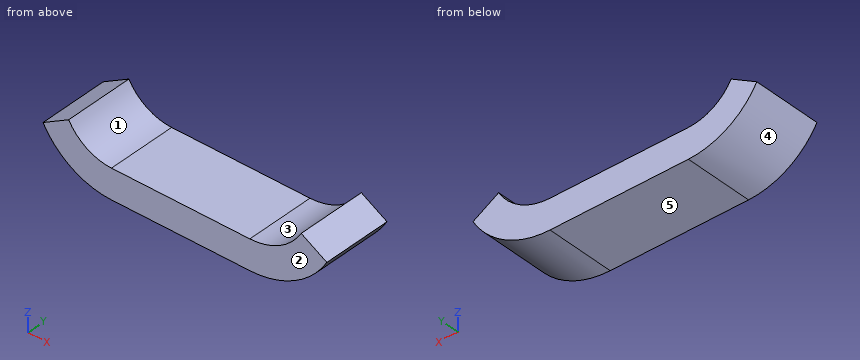
Autodesk Inventor part; units mm, degrees
ref_plane "YZ Plane" through (0, 0, 0) normal (1, 0, 0) x (0, 1, 0)
ref_plane "XZ Plane" through (0, 0, 0) normal (0, 1, 0) x (-1, 0, 0)
ref_plane "XY Plane" through (0, 0, 0) normal (0, 0, 1) x (1, 0, 0)
sketch "スケッチ1" plane through (0, 0, 0) normal (0, 1, 0) x (-1, 0, 0)
  circle A0 centre (70, -20) radius 80
  circle A1 centre (-70, -10) radius 90
  line L0 (70, -100) -> (-70, -100)
  line L1 (70, -20) -> (70, -100)
  line L2 (70, -20) -> (139.282, -60)
  line L3 (-70, -10) -> (-70, -100)
  line L4 (-70, -10) -> (-147.9423, -55)
  circle A2 centre (70, -20) radius 50
  circle A3 centre (-70, -10) radius 60
  line L5 (70, -70) -> (-70, -70)
  point P0 (0, 0)
  point P1 (113.3013, -45)
  point P2 (-121.9615, -40)
  dimension "d7" = 100
  dimension "d8" = 120
  dimension "d0" = 160
  dimension "d1" = 180
  dimension "d2" = 100
  dimension "d3" = 70
  dimension "d4" = 70
  dimension "d5" = 60
  dimension "d6" = 60
extrude "押し出し1" add sketch "スケッチ1" along normal mid plane 70 contours L1 A2 L2 A0 | L0 A1 L5 A0 | A0 L5 L1 | L3 L5 A1 | A1 L4 A3 L3
fillet "フィレット1" [suppressed]
properties part number "ArcSole2b"
Verification items for the finished model (mm, model axes). Face numbers are marked on the shaded views. A direction names the side the tool comes from. Give positions to 0.01 mm unless a question says otherwise; leave off trailing zeros. Order: outer loops, then holes, each group sorted by start corner. A loop starts at its lowest first (then second) coordinate and runs counter-clockwise, first axis right, second up. Notation, with made-up numbers: M -17.75,48.5 L 28.25,48.5 A6 cw 28.25,56.5 Z; hole C 58,80 d8. An arc over 180 degrees is marked long. Return JSON: item names as keys, results as strings. Group by question number.
1) Section check B-B on y = 17.5. Record the cut outline in (x, z), and give its area (3 significant figures).
2) Section check D-D on z = -73.5. Record the cut outline in (x, y), and give its area (3 significant figures).
3) Mould release check, pull along X, two halves, no side actions. Record for the marked faces 3, 4 and 5: pulls with the +X half, pulls with the -X half, needs draft (parallel to the pull), parting line crosses it, or undercut.
4) Access from +Z, -Z, +X, -X, +Y, -Y to the whole of each face (thin tool, end or side, straight path). Record for the marked faces 1 and 2.
5) Section check C-C on x = -9. Record the cut outline in (y, z).
6) Section check A-A on z = -57.5. Record the cut outline in (x, y).
7) Scan lines: line 1 (Z direction, x = 9, y = -5); line 2 (X direction, y = 29, z = -52); line 3 (X direction, y = 4, z = -71). Record each from-to range of solid material in increasing order.
8) Go/stop test with flat-tipped pins: pin 1 Ø1.5 at (y, z) = (-11.5, -56) entering from +X; pin 2 Ø1 at (x, y) = (-20.5, 26) entering from +Z. Record where each tip stops, or that it passes through.
Answer block:
{
 "1": {"outline": "M -139.28,-60 A80 ccw -70,-100 L 70,-100 A90 ccw 147.94,-55 L 121.96,-40 A60 cw 70,-70 L -70,-70 A50 cw -113.3,-45 Z", "area": "8,600 mm^2"},
 "2": {"outline": "M -129.48,-35 L 133.78,-35 L 133.78,35 L -129.48,35 Z", "area": "18,400 mm^2"},
 "3": {"face 3": "undercut", "face 4": "pulls with the -X half", "face 5": "needs draft"},
 "4": {"face 1": "+Z, +Y, -Y", "face 2": "+Z, -Z, +X, -X, -Y"},
 "5": {"outline": "M -35,-100 L 35,-100 L 35,-70 L -35,-70 Z"},
 "6": {"outline": "M -134.95,-35 L -103.07,-35 L -103.07,35 L -134.95,35 Z; M 106.66,-35 L 146.44,-35 L 146.44,35 L 106.66,35 Z"},
 "7": {"line 1": "z = -100 to -70", "line 2": "x = -125.43 to -108.42, 112.85 to 142.75", "line 3": "x = -131.64 to 136.17"},
 "8": {"pin 1": "stops at x = 147.8", "pin 2": "stops at z = -70"}
}
